Design review of the part built by this model. Coordinates are the model's own, in mm. Face numbers are marked on the shaded views. A direction names the side the tool comes from. Give positions to 0.01 mm unless a question says otherwise; leave off trailing zeros. Order: outer loops, then holes, each group sorted by start corner. A loop starts at its lowest first (then second) coordinate and runs counter-clockwise, first axis right, second up. Notation, with made-up numbers: M -2.5,57 L 4.5,57 A27 cw 4.5,84 Z; hole C 26.25,-30 d8. An arc over 180 degrees is marked long. Put each result on its own line as item: value. Start each with the question number.
from build123d import *

# Parameters (mm, degrees)
BOSS_EXTRUDE1_DEPTH = 24
CUT_EXTRUDE1_DEPTH  = 43
SKETCH4_R           = 12.7
CUT_EXTRUDE2_DEPTH  = 43
SKETCH5_R           = 5
CUT_EXTRUDE3_DEPTH  = 43
SKETCH6_R           = 7.5
SKETCH6_R_2         = 5
SKETCH6_R_3         = 30
SKETCH6_R_4         = 11
BOSS_EXTRUDE2_DEPTH = 1
SKETCH7_R           = 12.7
CUT_EXTRUDE4_DEPTH  = 10
CUT_EXTRUDE5_START  = -10
SKETCH8_R           = 12.7
CUT_EXTRUDE5_DEPTH  = 10


with BuildPart() as part:
    # Sketch1 → Boss-Extrude1 (new, symmetric)
    with BuildSketch(Plane.XY):
        with BuildLine():
            Line((0, 41.872855029), (0, -41.872855029))
            ThreePointArc((0, -41.872855029), (5.455474373, -55.600810969), (18.845677428, -61.839515726))
            Line((18.845677428, -61.839515726), (160, -70))
            ThreePointArc((160, -70), (230, 0), (160, 70))
            Line((160, 70), (18.845677428, 61.839515726))
            ThreePointArc((18.845677428, 61.839515726), (5.455474373, 55.600810969), (0, 41.872855029))
        make_face()
    extrude(amount=BOSS_EXTRUDE1_DEPTH, both=True)

    # Sketch2 → Cut-Extrude1 (cut)
    with BuildSketch(Plane(origin=(0, 0, -24), x_dir=(-1, 0, 0), z_dir=(0, 0, -1))):
        with BuildLine():
            Line((-19.134258071, 56.847850552), (-160.141737643, 64.999845465))
            ThreePointArc((-160.141737643, 64.999845465), (-225, 0), (-160.141737643, -64.999845465))
            Line((-160.141737643, -64.999845465), (-19.134258071, -56.847850552))
            ThreePointArc((-19.134258071, -56.847850552), (-9.09160578, -52.168821984), (-5, -41.872855029))
            Line((-5, -41.872855029), (-5, 41.872855029))
            ThreePointArc((-5, 41.872855029), (-9.09160578, 52.168821984), (-19.134258071, 56.847850552))
        make_face()
    extrude(amount=-CUT_EXTRUDE1_DEPTH, mode=Mode.SUBTRACT)

    # Sketch4 → Cut-Extrude2 (cut)
    with BuildSketch(Plane.XY.offset(24)):
        with Locations((160, 0)):
            Circle(SKETCH4_R)
    extrude(amount=-CUT_EXTRUDE2_DEPTH, mode=Mode.SUBTRACT)

    # Sketch5 → Cut-Extrude3 (cut)
    with BuildSketch(Plane.XY.offset(24)):
        with Locations((121, 35)):
            Circle(SKETCH5_R)
        with Locations((191, 35)):
            Circle(SKETCH5_R)
        with Locations(Location((191, -35, 0), (0, 0, 180))):
            Circle(SKETCH5_R)
        with Locations(Location((121, -35, 0), (0, 0, 180))):
            Circle(SKETCH5_R)
    extrude(amount=-CUT_EXTRUDE3_DEPTH, mode=Mode.SUBTRACT)

    # Sketch6 → Boss-Extrude2 (add, symmetric)
    # profile 1 of 5: a face of its own
    with BuildSketch(Plane.XY.offset(24)):
        with Locations((121, 35)):
            Circle(SKETCH6_R)
        with Locations((121, 35)):
            Circle(SKETCH6_R_2, mode=Mode.SUBTRACT)
    # profile 2 of 5: a face of its own
    with BuildSketch(Plane.XY.offset(24)):
        with Locations(Location((121, -35, 0), (0, 0, 180))):
            Circle(SKETCH6_R)
        with Locations(Location((121, -35, 0), (0, 0, 180))):
            Circle(SKETCH6_R_2, mode=Mode.SUBTRACT)
    # profile 3 of 5: a face of its own
    with BuildSketch(Plane.XY.offset(24)):
        with Locations(Location((191, 35, 0), (0, 0, 180))):
            Circle(SKETCH6_R)
        with Locations(Location((191, 35, 0), (0, 0, 180))):
            Circle(SKETCH6_R_2, mode=Mode.SUBTRACT)
    # profile 4 of 5: a face of its own
    with BuildSketch(Plane.XY.offset(24)):
        with Locations((191, -35)):
            Circle(SKETCH6_R)
        with Locations((191, -35)):
            Circle(SKETCH6_R_2, mode=Mode.SUBTRACT)
    # profile 5 of 5: a face of its own
    with BuildSketch(Plane.XY.offset(24)):
        with Locations((160, 0)):
            Circle(SKETCH6_R_3)
        with Locations((160, 0)):
            Circle(SKETCH6_R_4, mode=Mode.SUBTRACT)
    extrude(amount=BOSS_EXTRUDE2_DEPTH, both=True)

    # Sketch7 → Cut-Extrude4 (cut)
    with BuildSketch(Plane.XY.offset(24)):
        with Locations((50, 0)):
            Circle(SKETCH7_R)
    extrude(amount=-CUT_EXTRUDE4_DEPTH, mode=Mode.SUBTRACT)

    # Sketch8 → Cut-Extrude5 (cut)
    with BuildSketch(Plane(origin=(0, 0, 23), x_dir=(-1, 0, 0), z_dir=(0, 0, -1)).offset(CUT_EXTRUDE5_START)):
        with Locations(Location((-160, 0, 0), (0, 0, 180))):
            Circle(SKETCH8_R)
    extrude(amount=CUT_EXTRUDE5_DEPTH, mode=Mode.SUBTRACT)


solid = part.part
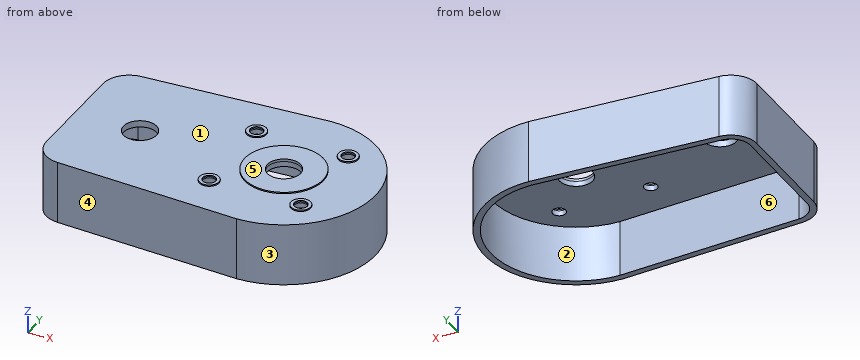
1. Consider section B-B on z = 11.5. Give the boundary of the cut face in (x, y).
2. Consider section D-D on x = 121. Give the boundary of the cut face in (y, z).
3. The part is to be moulded in two halves that separate along Y. For the marked faces 4, 5 and 6, say which applies: +Y half, -Y half, draft (parallel to the pull), parting line (faces both ways), or undercut.
4. Machinability: for the marked faces 1, 2 and 3, which of the approach directions +Z, -Z, +X, -X, +Y, -Y give a long, thin tool a straight path to every point of the face, cutting with its end or side? Answer none if there is none.
5. Consider section C-C on x = 42.5. Give the boundary of the cut face in (y, z).
6. Insertion check: pin 1 (10 mm diameter, centred on x = 43, z = 1.5, fed in from -Y) (3 decimals); pin 2 (16 mm diameter, centred on x = 191, y = -35, fed in from -Z); pin 3 (12 mm diameter, centred on y = -26.5, z = -6, fed in from +X). Each pin has a flat end and moves straight along its axis. Give the tip position at first contact, or say it passes through.
7. Consider section A-A on y = 0. Give the boundary of the cut face in (x, z).
8. To check wall thickness, follow probe 1 along Y at (x, z) = (191, 19.9); probe 2 along X at (y, z) = (1, 11); probe 3 along Y at (x, z) = (121, 21). State the ranges of each line that lie inside material, in increasing order.
Returned:
1. outline: M 0,-41.87 A20 ccw 18.85,-61.84 L 160,-70 A70 ccw 160,70 L 18.85,61.84 A20 ccw 0,41.87 Z; hole M 5,-41.87 A15 ccw 19.13,-56.85 L 160.14,-65 A65 ccw 160.14,65 L 19.13,56.85 A15 ccw 5,41.87 Z
2. outline: M -67.75,-24 L -62.74,-24 L -62.74,19 L -40,19 L -40,25 L -42.5,25 L -42.5,24 L -67.75,24 Z; M -30,19 L 30,19 L 30,25 L 27.5,25 L 27.5,24 L -27.5,24 L -27.5,25 L -30,25 Z; M 40,19 L 62.74,19 L 62.74,-24 L 67.75,-24 L 67.75,24 L 42.5,24 L 42.5,25 L 40,25 Z
3. face 4: -Y half
3. face 5: draft
3. face 6: undercut
4. face 1: +Z
4. face 2: -Z
4. face 3: +Z, -Z, +X
5. outline: M -63.21,-24 L -58.2,-24 L -58.2,19 L -10.25,19 L -10.25,24 L -63.21,24 Z; M 10.25,19 L 58.2,19 L 58.2,-24 L 63.21,-24 L 63.21,24 L 10.25,24 Z
6. pin 1: stops at y = -63.525
6. pin 2: stops at z = 19
6. pin 3: stops at x = 226.93
7. outline: M 0,-24 L 5,-24 L 5,19 L 37.3,19 L 37.3,24 L 0,24 Z; M 62.7,19 L 147.3,19 L 147.3,25 L 130,25 L 130,24 L 62.7,24 Z; M 172.7,19 L 225,19 L 225,-24 L 230,-24 L 230,24 L 190,24 L 190,25 L 172.7,25 Z
8. probe 1: y = -62.76 to -40, -30 to 30, 40 to 62.76
8. probe 2: x = 0 to 5, 224.99 to 229.99
8. probe 3: y = -67.75 to -40, -30 to 30, 40 to 67.75
